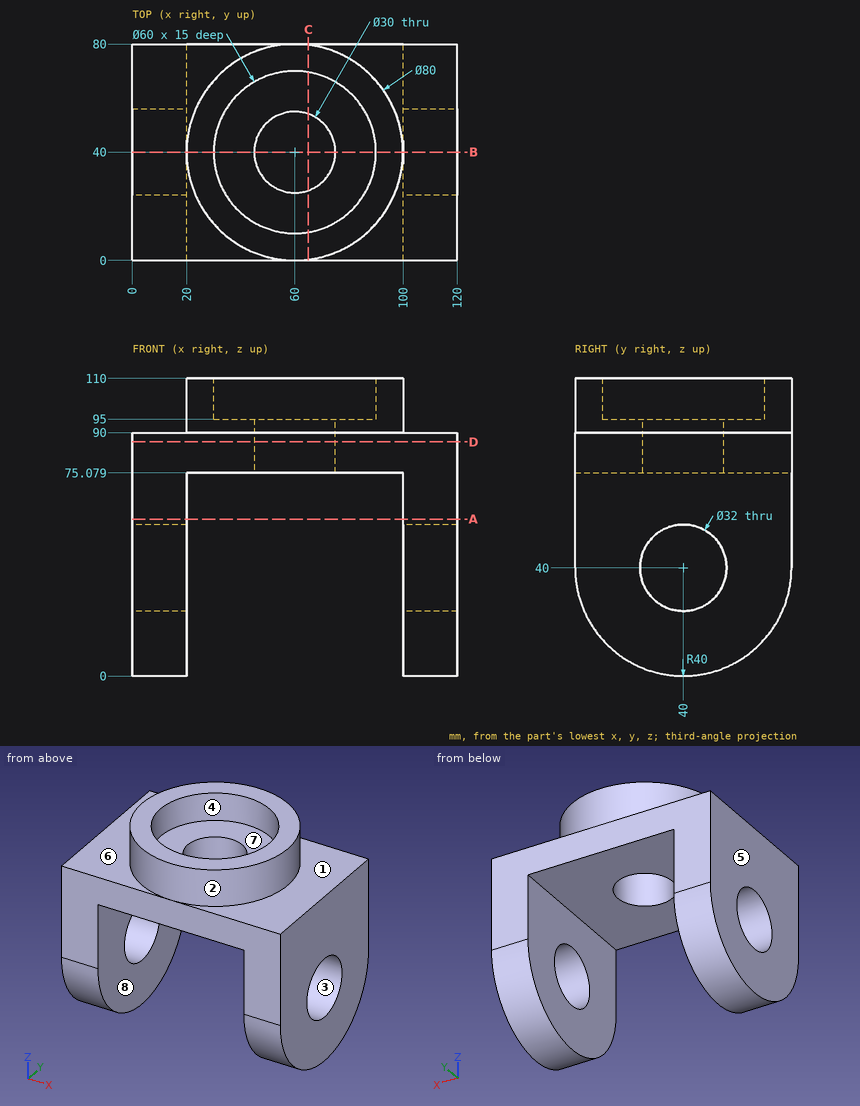
For this review, use the dimensioned drawing (mm, ordinates from the lowest corner) and the shaded views. A direction names the side the tool comes from. Coordinates: 2 decimals unless noted, no trailing zeros. Loops run counter-clockwise (first coordinate to the right, second up) from the corner with the lowest first, then second, coordinate; pieces in that order, holes last. Notation, with made-up numbers: (-30.75, 72.5) - (-8.75, 72.5) arc R27 cw to (-8.75, 96.5) - close; hole circle Ø7 at (65, 13). An arc over 180 degrees is marked (long way). Use CSV: the item, a comma, the result in double quotes. Start each with the question number.
1) For pin 1 Ø10 at (x, z) = (31.5, 98) entering from -Y; pin 2 Ø18 at (x, y) = (17, 28.5) entering from +Z; pin 3 Ø5 at (x, z) = (107.5, 93.5) entering from -Y, all flat-tipped, find the tip position at first contact; note any pin that passes through.
2) Consider section C-C on x = 65. Write out the cut boundary in (y, z).
3) Consider section A-A on z = 58. Write out the cut boundary in (x, y).
4) Consider section B-B on y = 40. Write out the cut boundary in (x, z), then the cut area to 3 significant figures.
5) Consider section D-D on z = 86.5. Write out the cut boundary in (x, y), then the cut area to 3 significant figures.
6) The part is to be moulded in two halves that separate along Y. For the marked faces 1, 2, 3 and 4, say which applies: +Y half, -Y half, draft (parallel to the pull), parting line (faces both ways), or undercut.
7) Tool access review of the marked faces 5, 6, 7 and 8: name each direction out of +Z, -Z, +X, -X, +Y, -Y from which nothing blocks a thin tool from reaching the whole face with its end or side.
8) Wall thickness on L1, parallel to Y at x = 60, z = 102; L2, parallel to Y at x = 60, z = 84.75; L3, parallel to X at y = 54, z = 73: over which ranges is each line inside the solid? List them lowest first. Write a range as from..to.
Geometry says:
1,pin 1,"y = 7.63"
1,pin 2,"z = 110"
1,pin 3,"through"
2,outline,"(0, 75.08) - (25.86, 75.08) - (25.86, 95) - (10.42, 95) - (10.42, 110) - (0.31, 110) - (0.31, 90) - (0, 90) - close; (54.14, 75.08) - (80, 75.08) - (80, 90) - (79.69, 90) - (79.69, 110) - (69.58, 110) - (69.58, 95) - (54.14, 95) - close"
3,outline,"(0, 0) - (20, 0) - (20, 80) - (0, 80) - close; (100, 0) - (120, 0) - (120, 80) - (100, 80) - close"
4,outline,"(0, 0) - (20, 0) - (20, 24) - (0, 24) - close; (0, 56) - (20, 56) - (20, 75.08) - (45, 75.08) - (45, 95) - (30, 95) - (30, 110) - (20, 110) - (20, 90) - (0, 90) - close; (75, 75.08) - (100, 75.08) - (100, 56) - (120, 56) - (120, 90) - (100, 90) - (100, 110) - (90, 110) - (90, 95) - (75, 95) - close; (100, 0) - (120, 0) - (120, 24) - (100, 24) - close"
4,area,"3,620 mm^2"
5,outline,"(0, 0) - (120, 0) - (120, 80) - (0, 80) - close; hole circle Ø30 at (60, 40)"
5,area,"8,890 mm^2"
6,face 1,"draft"
6,face 2,"parting line"
6,face 3,"undercut"
6,face 4,"undercut"
7,face 5,"+Z, -Z, -X, +Y, -Y"
7,face 6,"+Z, -X"
7,face 7,"+Z"
7,face 8,"-Z, +Y, -Y"
8,L1,"0..10, 70..80"
8,L2,"0..25, 55..80"
8,L3,"0..20, 100..120"
